```python
from build123d import *

# Parameters (mm, degrees)
SKETCH1_W                        = 6.35
SKETCH1_H                        = 31.75
SKETCH1_W_2                      = 69.85
SKETCH1_H_2                      = 12.7
F_1_2_20_TAPPED_HOLE1_D          = 11.50874
SKETCH7_W                        = 2.5527
SKETCH7_H                        = 87.122
F_1_4_20_TAPPED_HOLE1_AT_2_COUNT = 2
F_1_4_20_TAPPED_HOLE1_AT_2_PITCH = 12.7


with BuildPart() as part:
    # Sketch1 → Revolve1 (revolve)
    with BuildSketch(Plane.XY, mode=Mode.PRIVATE) as revolve1_sk:
        with Locations((20.447, 28.575)):
            Rectangle(SKETCH1_W, SKETCH1_H)
        with Locations((52.197, 6.35)):
            Rectangle(SKETCH1_W_2, SKETCH1_H_2)
    revolve(revolve1_sk.sketch.rotate(Axis((0, 7.809475806, 0), (0, -1, 0)), 90), axis=Axis((0, 7.809475806, 0), (0, -1, 0)))

    # 1/2-20 Tapped Hole1 (through all)
    with Locations(Plane(origin=(0, 12.7, 0), x_dir=(1, 0, 0), z_dir=(0, 1, 0))):
        with Locations((-54.155626078, 18.25625), (0, 57.15), (54.155626078, 18.25625), (34.599427772, -45.486284722), (-34.599427772, -45.486284722)):
            Hole(F_1_2_20_TAPPED_HOLE1_D / 2)

    # Sketch7 → 1/4-20 Tapped Hole1 (revolve, cut)
    with BuildSketch(Plane.ZX.offset(38.1)):
        with Locations((1.27635, 43.561)):
            Rectangle(SKETCH7_W, SKETCH7_H)
    f_1_4_20_tapped_hole1 = revolve(axis=Axis((-6.35, 38.1, 0), (1, 0, 0)), mode=Mode.SUBTRACT)

    # 1/4-20 Tapped Hole1 at 2: 1/4-20 Tapped Hole1 ×2
    with Locations(*[(0, -i * F_1_4_20_TAPPED_HOLE1_AT_2_PITCH, 0) for i in range(1, F_1_4_20_TAPPED_HOLE1_AT_2_COUNT)]):
        add(f_1_4_20_tapped_hole1, mode=Mode.SUBTRACT)


solid = part.part
```
Model file for the job. Use its own axes, mm. A direction names the side the tool comes from. Coordinates: 2 decimals unless noted, no trailing zeros. Loops run counter-clockwise (first coordinate to the right, second up) from the corner with the lowest first, then second, coordinate; pieces in that order, holes last. Notation, with made-up numbers: (8.5, 69) - (52.5, 69) arc R11 cw to (52.5, 86) - close; hole circle Ø7 at (43.25, 59.25). An arc over 180 degrees is marked (long way). Answer as a JSON object with one key per item and string values. Group by question number.
(1) Cut at B-B (x = -50.5). Give the cut face in (y, z), then the cut area to 3 significant figures.
(2) Cut at A-A (z = 0). Give the cut face in (x, y), then the cut area to 3 significant figures.
(3) Cut at D-D (z = -57.15). Give the cut face in (x, y), then the cut area to 3 significant figures.
(4) Flat gauge pins, fed straight in: pin 1 (5 mm diameter, centred on y = 4.5, z = -60, fed in from +X); pin 2 (1 mm diameter, centred on x = 10.5, y = 18.5, fed in from -Z); pin 3 (20.5 mm diameter, centred on x = 0, z = 0, fed in from +Y); pin 4 (2 mm diameter, centred on x = 10, y = 6, fed in from -Z). Where does each tip first touch, or does it go through?
(5) Cut at C-C (y = 17). Give the cut face in (x, z).
(6) Tool access for faces 1 (the face through (20.4, 26.95, -2.03)), 2 (the face through (17.4, 44.45, -1.6)), 3 (the face through (14.37, 28.8, -18.75)): list every direction of +Z, -Z, +X, -X, +Y, -Y with a clear straight run to the whole face (end or side of a thin tool).
(7) Two-plate mould, pull along X, no slides. Class faces 4 (the face through (18, 0, 1)), 5 (the face through (39.166, 6.261, 48.988)), 6 (the face through (-86.38, 6.44, -11.34)): released by +X, released by -X, zero draft, split by the parting line, or undercut.
(8) Probe line 1 along Y through (x, z) = (20.75, 0); line 2 along X through (y, z) = (10, 41); line 3 along Y through (x, z) = (59.5, 43.5). List the from-to ranges inside material, lowest first.
Geometry says:
{
 "1": {"outline": "(0, -70.99) - (12.7, -70.99) - (12.7, -22.7) - (0, -22.7) - close; (0, -13.81) - (12.7, -13.81) - (12.7, 70.99) - (0, 70.99) - close", "area": "1,690 mm^2"},
 "2": {"outline": "(-87.12, 0) - (-17.27, 0) - (-17.27, 44.45) - (-23.62, 44.45) - (-23.62, 12.7) - (-87.12, 12.7) - close; (17.27, 0) - (87.12, 0) - (87.12, 12.7) - (23.62, 12.7) - (23.62, 22.85) - (17.27, 22.85) - close; (17.27, 27.95) - (23.62, 27.95) - (23.62, 35.55) - (17.27, 35.55) - close; (17.27, 40.65) - (23.62, 40.65) - (23.62, 44.45) - (17.27, 44.45) - close", "area": "2,110 mm^2"},
 "3": {"outline": "(-65.76, 0) - (-5.75, 0) - (-5.75, 12.7) - (-65.76, 12.7) - close; (5.75, 0) - (65.76, 0) - (65.76, 12.7) - (5.75, 12.7) - close", "area": "1,520 mm^2"},
 "4": {"pin 1": "stops at x = 65.45", "pin 2": "stops at z = -21.4", "pin 3": "passes through", "pin 4": "stops at z = -86.66"},
 "5": {"outline": "circle Ø47.24 at (0, 0); hole circle Ø34.54 at (0, 0)"},
 "6": {"face 1": "+X", "face 2": "+Z, -Z, +X, -X, +Y", "face 3": "+Y"},
 "7": {"face 4": "zero draft", "face 5": "undercut", "face 6": "split by the parting line"},
 "8": {"line 1": "y = 0 to 22.85, 27.95 to 35.55, 40.65 to 44.45", "line 2": "x = -76.87 to -38.2, -31 to 31, 38.2 to 76.87", "line 3": "y = 0 to 12.7"}
}
